The listing builds one solid part. Answer for the finished solid, in the listing's coordinates (mm). Face numbers are marked on the shaded views. Coordinates: 2 decimals unless noted, no trailing zeros. Loops run counter-clockwise (first coordinate to the right, second up) from the corner with the lowest first, then second, coordinate; pieces in that order, holes last. Notation, with made-up numbers: M 60.25,58 L 75.25,58 A28 cw 75.25,80 Z; hole C 64,22 d9. An arc over 180 degrees is marked long. Answer as CSV lines item,"result". Start each with the question number.
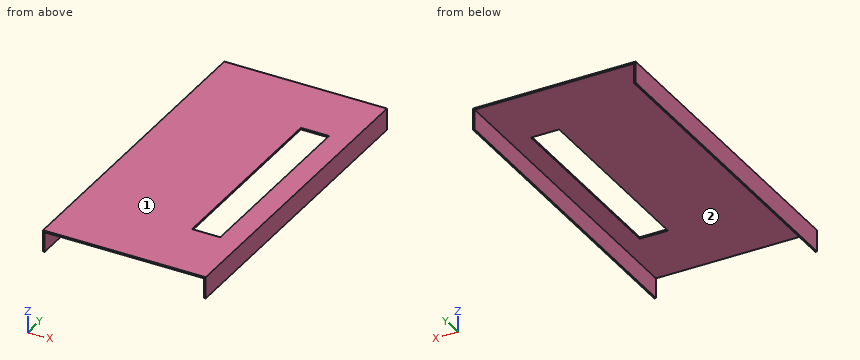
```python
from build123d import *

# Parameters (mm, degrees)
OVEN_YAG_KABI_KAPAGI_KAPAK_1_START = 820
OVEN_YAG_KABI_KAPAGI_KAPAK_1_DEPTH = 300
OVEN_YAG_KABI_KAPAGI_KAPAK_2_START = 27
SKETCH2_W                          = 26
SKETCH2_H                          = 180
OVEN_YAG_KABI_KAPAGI_KAPAK_2_DEPTH = 14


with BuildPart() as part:
    # Sketch1 → OVEN_yag_kabi_kapagi_kapak_1 (new body)
    with BuildSketch(Plane(origin=(0, 0, 0), x_dir=(1, 0, 0), z_dir=(0, 1, 0)).offset(OVEN_YAG_KABI_KAPAGI_KAPAK_1_START)):
        Polygon((30, -40), (30, -20), (31.5, -20), (31.5, -38.5), (178.5, -38.5), (178.5, -20), (180, -20), (180, -40), align=None)
    extrude(amount=OVEN_YAG_KABI_KAPAGI_KAPAK_1_DEPTH)

    # Sketch2 → OVEN_yag_kabi_kapagi_kapak_2 (cut)
    with BuildSketch(Plane.XY.offset(OVEN_YAG_KABI_KAPAGI_KAPAK_2_START)):
        with Locations((147, 970)):
            Rectangle(SKETCH2_W, SKETCH2_H)
    extrude(amount=OVEN_YAG_KABI_KAPAGI_KAPAK_2_DEPTH, mode=Mode.SUBTRACT)


solid = part.part
```
Item 1: For a pull along X with two mould halves and no side action, classify the marked faces 1 and 2 as pulls with the +X half, pulls with the -X half, needs draft (parallel to the pull), parting line crosses it, or undercut.
Item 2: Section C-C on z = 32.5 is taken. Determine the outline of the cut face in (x, y), then the cut area to 3 significant figures.
Item 3: Section D-D on y = 1092 is taken. Determine the outline of the cut face in (x, z).
Item 4: Section A-A on y = 911.5 is taken. Determine the outline of the cut face in (x, z), then the cut area to 4 significant figures.
Item 5: Consider line 1 (X direction, y = 893, z = 33.5); line 2 (Z direction, x = 123.5, y = 992.5). Determine where each line is inside the solid, lowest interval first.
Item 6: Each of these flat-tipped pins is pushed along its axis until it touches: P1, Ø12, axis at x = 148.5, y = 976.5, coming from the -Z side; P2, Ø4, axis at x = 50.5, y = 1024.5, coming from the -Z side. Where does it stop, or does it pass through?
Item 7: Section B-B on x = 143.5 is taken. Determine the outline of the cut face in (y, z).
Results are:
1,face 1,"needs draft"
1,face 2,"undercut"
2,outline,"M 30,820 L 31.5,820 L 31.5,1120 L 30,1120 Z; M 178.5,820 L 180,820 L 180,1120 L 178.5,1120 Z"
2,area,"900 mm²"
3,outline,"M 30,20 L 31.5,20 L 31.5,38.5 L 178.5,38.5 L 178.5,20 L 180,20 L 180,40 L 30,40 Z"
4,outline,"M 30,20 L 31.5,20 L 31.5,38.5 L 134,38.5 L 134,40 L 30,40 Z; M 160,38.5 L 178.5,38.5 L 178.5,20 L 180,20 L 180,40 L 160,40 Z"
4,area,"241.5 mm²"
5,line 1,"30 to 31.5, 178.5 to 180"
5,line 2,"38.5 to 40"
6,P1,"through"
6,P2,"z = 38.5"
7,outline,"M 820,38.5 L 880,38.5 L 880,40 L 820,40 Z; M 1060,38.5 L 1120,38.5 L 1120,40 L 1060,40 Z"
